Check sheet for the modelled part. Datum: model origin and axes. Units: mm. A direction names the side the tool comes from. Round coordinates to 2 decimals unless told otherwise and drop trailing zeros. Write each loop counter-clockwise with the first axis right and the second up, starting at its lowest first coordinate (ties: lowest second). Pieces come first, ordered by that corner, then holes. Notation, with made-up numbers: (6.25, 31.5) - (14.25, 31.5) arc R29 ccw to (14.25, 66.5) - close; hole circle Ø1 at (-32.75, 5). An arc over 180 degrees is marked (long way). Use one line per item in the form item = value. Start each with the question number.
1) Draft check along Z on faces 6 (the face through (2, 38.1, 10)), 7 (the face through (21.4, 38.88, 7.18)), 8 (the face through (28.894, 19.566, 9.53)). Enter one of: +Z half, -Z half, draft (parallel to the pull), parting line (faces both ways), or undercut.
2) Gauge pin test, flat ends, axial feed: P1, Ø10, axis at y = 8.5, z = 4.5, coming from the +X side; P2, Ø5.5, axis at x = 8, z = 10.5, coming from the -Y side; P3, Ø1.3, axis at y = 39, z = 17.5, coming from the +X side; P4, Ø21, axis at x = 15, y = 14.5, coming from the +Z side. Record the tip position at first contact, or that the pin passes through.
3) Section check A-A (x = 24). Record the boundary of the cut face in (y, z), then the cut area to 3 significant figures.
4) Section check D-D (y = 20). Count the separate pieces of the cut face and the enclosed holes in it, then the cut area to 3 significant figures.
5) Scan lines: probe 1 along X at (y, z) = (18, 10.25); probe 2 along X at (y, z) = (31.5, 5); probe 3 along X at (y, z) = (14, 6.5). Record each from-to range of solid material in increasing order.
6) Set-up check for faces 1 (the face through (18, 21, 15.74)), 2 (the face through (-13.638, 19, 17)), 3 (the face through (17.788, 18.783, 9.181)), 4 (the face through (-18, 20, 18.915)), 5 (the face through (16.609, 19, 14)): record each of +Z, -Z, +X, -X, +Y, -Y from which the full face is reachable in a straight line by a thin tool's end or side.
7) Section check C-C (x = 6). Record the boundary of the cut face in (y, z), then the cut area to 3 significant figures.
8) Section check B-B (z = 3.75). Record the boundary of the cut face in (x, y).
from build123d import *

# Parameters (mm, degrees)
SKETCH2_R           = 4.7625
BOSS_EXTRUDE1_DEPTH = 38.1
SKETCH3_R           = 2.4892
BOSS_EXTRUDE2_DEPTH = 1.5875
SKETCH4_W           = 20.112893425
SKETCH4_H           = 3.175
SKETCH4_W_2         = 10.134015187
BOSS_EXTRUDE3_DEPTH = 1.5875
FILLET2_R           = 6.35


with BuildPart() as part:
    # Sketch2 → Boss-Extrude1 (new body)
    with BuildSketch(Plane(origin=(0, 0, 0), x_dir=(1, 0, 0), z_dir=(0, 1, 0))):
        with BuildLine():
            Line((-13.637822674, -18.9154966), (-13.637822674, -15.7404966))
            ThreePointArc((-13.637822674, -15.7404966), (0, 0), (16.609085938, -12.5654966))
            Line((16.609085938, -12.5654966), (16.609085938, -15.7404966))
            Line((16.609085938, -15.7404966), (22.545691393, -15.7404966))
            ThreePointArc((22.545691393, -15.7404966), (28.895691393, -9.3904966), (22.545691393, -3.0404966))
            ThreePointArc((22.545691393, -3.0404966), (18.914562129, -2.601594541), (15.492581173, -1.310168551))
            ThreePointArc((15.492581173, -1.310168551), (-2.207478742, 2.815047226), (-17.640279185, -6.783817119))
            ThreePointArc((-17.640279185, -6.783817119), (-18.810770101, -6.984553123), (-19.996688426, -7.047335697))
            ThreePointArc((-19.996688426, -7.047335697), (-26.135207048, -11.772192893), (-23.138726022, -18.9154966))
            Line((-23.138726022, -18.9154966), (-13.637822674, -18.9154966))
        make_face()
        with Locations((-19.996688426, -13.397335697)):
            Circle(SKETCH2_R, mode=Mode.SUBTRACT)
        with Locations((22.545691393, -9.3904966)):
            Circle(SKETCH2_R, mode=Mode.SUBTRACT)
    extrude(amount=BOSS_EXTRUDE1_DEPTH)

    # Sketch3 → Boss-Extrude2 (add)
    with BuildSketch(Plane(origin=(0, 38.1, 0), x_dir=(-1, 0, 0), z_dir=(0, 1, 0))):
        with BuildLine():
            Line((13.637822674, 15.7404966), (3.503807487, 15.7404966))
            Line((3.503807487, 15.7404966), (3.503807487, 12.5654966))
            Line((3.503807487, 12.5654966), (-16.609085938, 12.5654966))
            Line((-16.609085938, 12.5654966), (-16.609085938, 15.7404966))
            Line((-16.609085938, 15.7404966), (-22.545691393, 15.7404966))
            ThreePointArc((-22.545691393, 15.7404966), (-28.895691393, 9.3904966), (-22.545691393, 3.0404966))
            ThreePointArc((-22.545691393, 3.0404966), (-18.914562129, 2.601594541), (-15.492581173, 1.310168551))
            ThreePointArc((-15.492581173, 1.310168551), (2.207478742, -2.815047226), (17.640279185, 6.783817119))
            ThreePointArc((17.640279185, 6.783817119), (18.810770101, 6.984553123), (19.996688426, 7.047335697))
            ThreePointArc((19.996688426, 7.047335697), (26.135207048, 11.772192893), (23.138726022, 18.9154966))
            Line((23.138726022, 18.9154966), (13.637822674, 18.9154966))
            Line((13.637822674, 18.9154966), (13.637822674, 15.7404966))
        make_face()
        with Locations((-22.545691393, 9.3904966)):
            Circle(SKETCH3_R, mode=Mode.SUBTRACT)
        with Locations((19.996688426, 13.397335697)):
            Circle(SKETCH3_R, mode=Mode.SUBTRACT)
    extrude(amount=BOSS_EXTRUDE2_DEPTH)

    # Sketch4 → Boss-Extrude3 (add)
    with BuildSketch(Plane(origin=(0, 39.6875, 0), x_dir=(-1, 0, 0), z_dir=(0, 1, 0))):
        with Locations((-6.552639226, 14.1529966)):
            Rectangle(SKETCH4_W, SKETCH4_H)
        with Locations((8.570815081, 17.3279966)):
            Rectangle(SKETCH4_W_2, SKETCH4_H)
    extrude(amount=-BOSS_EXTRUDE3_DEPTH)

    # Fillet2
    fillet2_edges = [part.edges().sort_by_distance(p)[0] for p in [
        (15.492581173, 19.84375, 1.310168551),
        (-17.640279185, 19.84375, 6.783817119),
    ]]
    fillet(fillet2_edges, radius=FILLET2_R)


solid = part.part
Results are:
q1.face_6 = draft
q1.face_7 = undercut
q1.face_8 = parting line
q2.P1 = 28.9
q2.P2 = 38.1
q2.P3 = -3.5
q2.P4 = 15.74
q3.outline = (0, 3.21) - (39.69, 3.21) - (39.69, 7.37) - (38.1, 7.37) - (38.1, 4.86) - (0, 4.86) - close; (0, 13.93) - (38.1, 13.93) - (38.1, 11.41) - (39.69, 11.41) - (39.69, 15.57) - (0, 15.57) - close
q3.area = 139 mm²
q4.separate_pieces = 1
q4.enclosed_holes = 2
q4.area = 284 mm²
q5.probe_1 = -25.51 to -23.57, -16.42 to -12.84, 16.02 to 17.86, 27.23 to 28.84
q5.probe_2 = -16.23 to -9.77, 12.95 to 20.7, 24.39 to 27.13
q5.probe_3 = -18.28 to -10.95, 14.13 to 18.76, 26.33 to 28.2
q6.face_1 = +Z, +X, +Y, -Y
q6.face_2 = +Z, +X, -Y
q6.face_3 = -Y
q6.face_4 = +Z, +X, -X, +Y, -Y
q6.face_5 = +Z, -Y
q7.outline = (0, -2.73) - (39.69, -2.73) - (39.69, 15.74) - (38.1, 15.74) - (38.1, 0.57) - (0, 0.57) - close
q7.area = 155 mm²
q8.outline = (-15.06, 0) - (-8.52, 0) - (-8.52, 38.1) - (11.7, 38.1) - (11.7, 0) - (25.46, 0) - (25.46, 39.69) - (-15.06, 39.69) - close
